from build123d import *

# Parameters (mm, degrees)
BOSS_EXTRUDE1_DEPTH                              = 440
CUT_EXTRUDE1_DEPTH                               = 441.332899634
CBORE_FOR_M4_HEX_HEAD_MACHINE_SCREW1_D           = 4.5
CBORE_FOR_M4_HEX_HEAD_MACHINE_SCREW1_DEPTH       = 15
CBORE_FOR_M4_HEX_HEAD_MACHINE_SCREW1_CBORE_D     = 7.5
CBORE_FOR_M4_HEX_HEAD_MACHINE_SCREW1_CBORE_DEPTH = 6
CHAMFER1_SIZE                                    = 0.75
CHAMFER2_SIZE                                    = 1.060660172


with BuildPart() as part:
    # Sketch1 → Boss-Extrude1 (new body)
    with BuildSketch(Plane(origin=(250, 0, 0), x_dir=(0, 0, -1), z_dir=(1, 0, 0))):
        Polygon((-7.5, 6), (-7.5, 0), (7.5, 0), (7.5, 6), (6, 7.5), (6, 10.5), (8.25, 12.75), (6, 15), (-6, 15), (-8.25, 12.75), (-6, 10.5), (-6, 7.5), align=None)
    extrude(amount=-BOSS_EXTRUDE1_DEPTH)

    # Sketch2 → Cut-Extrude1 (cut, through all)
    with BuildSketch(Plane.ZY.offset(190)):
        Polygon((-2.25, 0), (2.25, 0), (1.5, 0.75), (-1.5, 0.75), align=None)
    extrude(amount=-CUT_EXTRUDE1_DEPTH, mode=Mode.SUBTRACT)

    # CBORE for M4 Hex Head Machine Screw1
    with Locations(Plane(origin=(0, 15, 0), x_dir=(1, 0, 0), z_dir=(0, 1, 0))):
        with Locations((210, 0), (150, 0), (90, 0), (30, 0), (-30, 0), (-90, 0), (-150, 0), (-210, 0)):
            CounterBoreHole(CBORE_FOR_M4_HEX_HEAD_MACHINE_SCREW1_D / 2, CBORE_FOR_M4_HEX_HEAD_MACHINE_SCREW1_CBORE_D / 2, CBORE_FOR_M4_HEX_HEAD_MACHINE_SCREW1_CBORE_DEPTH, depth=CBORE_FOR_M4_HEX_HEAD_MACHINE_SCREW1_DEPTH)

    # Chamfer1
    chamfer1_edges = [part.edges().sort_by_distance(p)[0] for p in [
        (30, 0, -7.5),
        (30, 0, 7.5),
    ]]
    chamfer(chamfer1_edges, length=CHAMFER1_SIZE)

    # Chamfer2
    chamfer2_edges = [part.edges().sort_by_distance(p)[0] for p in [
        (30, 12.75, 8.25),
        (30, 12.75, -8.25),
    ]]
    chamfer(chamfer2_edges, length=CHAMFER2_SIZE)


solid = part.part
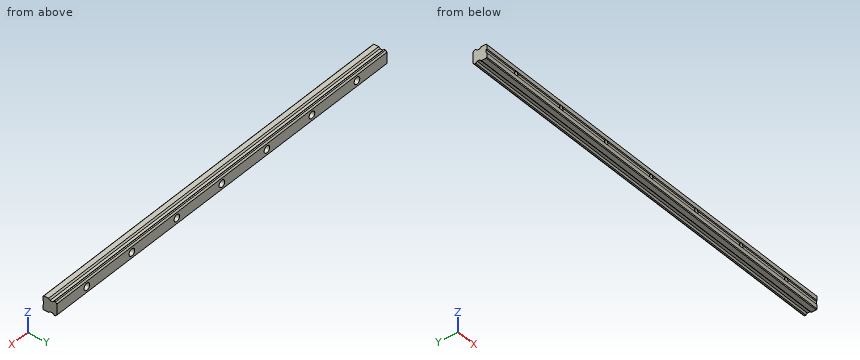
Design review of the part built by this model. Coordinates are the model's own, in mm. Coordinates: 2 decimals unless noted, no trailing zeros. Write each loop counter-clockwise with the first axis right and the second up, starting at its lowest first coordinate (ties: lowest second). Pieces come first, ordered by that corner, then holes. Notation, with made-up numbers: (62, 3.25) - (117, 3.25) arc R11 ccw to (117, 16.25) - close; hole circle Ø5 at (19.5, -38.75). An arc over 180 degrees is marked (long way). Use one line per item in the form item = value.
Q1. Consider section A-A (x = 125). Write out the cut boundary in (y, z), plus the area to 3 significant figures.
Taken from the geometry:
outline = (0, -6.75) - (0.75, -7.5) - (6, -7.5) - (7.5, -6) - (10.5, -6) - (12, -7.5) - (13.5, -7.5) - (15, -6) - (15, 6) - (13.5, 7.5) - (12, 7.5) - (10.5, 6) - (7.5, 6) - (6, 7.5) - (0.75, 7.5) - (0, 6.75) - (0, 2.25) - (0.75, 1.5) - (0.75, -1.5) - (0, -2.25) - close
area = 206 mm^2
Q2. Insertion check: pin 1 Ø2.5 at (x, z) = (210, 0) entering from +Y; pin 2 Ø1.5 at (x, y) = (39.5, 9) entering from -Z; pin 3 Ø3.5 at (x, z) = (-179.5, 0) entering from -Y; pin 4 Ø3.5 at (x, y) = (46.5, 9) entering from +Z. Each pin has a flat end and moves straight along its axis. Give the tip position at first contact, or say it passes through.
Taken from the geometry:
pin_1 = through
pin_2 = -6
pin_3 = 0.5
pin_4 = 6.25
Q3. For probe 1 along Z at (x, y) = (-30, 2.75); probe 2 along Y at (x, z) = (-32.5, 2.25); probe 3 along Z at (x, y) = (30, 7), list the stretches that pass through material, from the lowest coordinate up.
Taken from the geometry:
probe_1 = -7.5 to -2.25, 2.25 to 7.5
probe_2 = 0 to 9
probe_3 = -6.5 to -2.25, 2.25 to 6.5
